Answer from the drawing. Dimensions are ordinates in mm from the lowest x, y and z of the part. A direction names the side the tool comes from. Coordinates: 2 decimals unless noted, no trailing zeros. Order: outer loops, then holes, each group sorted by start corner. A loop starts at its lowest first (then second) coordinate and runs counter-clockwise, first axis right, second up.
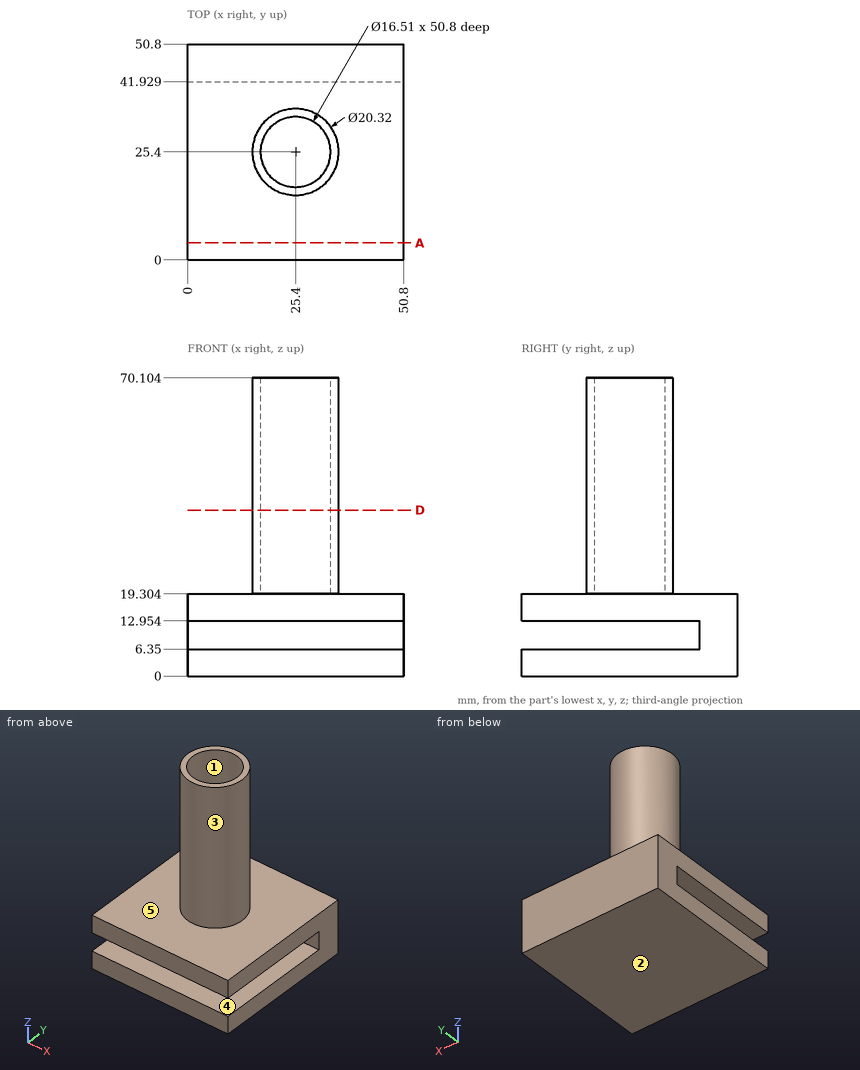
1. Flat-ended cylindrical pins translate along their axes: pin 1 (15 mm diameter, centred on x = 25.4, y = 25.4, fed in from -Z); pin 2 (10 mm diameter, centred on x = 34.5, z = 40.5, fed in from +Y); pin 3 (1 mm diameter, centred on y = 24.5, z = 35, fed in from -X); pin 4 (12 mm diameter, centred on x = 42.5, y = 33, fed in from +Z). Find the tip coordinate at first contact, or state that the pin passes through.
2. The part is cut by section D-D (z = 39). Determine the outline of the cut face in (x, y) (1 decimal).
3. For the marked faces 1 and 2, determine the directions among +Z, -Z, +X, -X, +Y, -Y from which every point of the face is accessible in a straight line to the end or side of a thin tool.
4. Consider probe 1 along Z at (x, y) = (28, 34.5); probe 2 along Y at (x, z) = (25, 40) (1 decimal); probe 3 along Y at (x, z) = (25.4, 41) (1 decimal). Determine where each line is inside the solid, lowest interval first.
5. The mould has two halves that part along Z. Classify the marked faces 3, 4 and 5: released by +Z, released by -Z, zero draft, split by the parting line, or undercut.
6. The part is cut by section A-A (y = 4). Determine the outline of the cut face in (x, z).
Worked out:
1. pin 1: stops at z = 0
1. pin 2: stops at y = 34.7
1. pin 3: stops at x = 15.25
1. pin 4: stops at z = 19.3
2. outline: circle Ø20.3 at (25.4, 25.4); hole circle Ø16.5 at (25.4, 25.4)
3. face 1: +Z
3. face 2: -Z, +X, -X, +Y, -Y
4. probe 1: z = 0 to 6.35, 12.95 to 70.1
4. probe 2: y = 15.2 to 17.2, 33.6 to 35.6
4. probe 3: y = 15.2 to 17.1, 33.7 to 35.6
5. face 3: zero draft
5. face 4: undercut
5. face 5: released by +Z
6. outline: (0, 0) - (50.8, 0) - (50.8, 6.35) - (0, 6.35) - close; (0, 12.95) - (50.8, 12.95) - (50.8, 19.3) - (0, 19.3) - close
